```python
from build123d import *

# Parameters (mm, degrees)
SKETCH1_W           = 195.38
SKETCH1_H           = 100
BOSS_EXTRUDE1_DEPTH = 3
SKETCH2_R           = 2.75
CUT_EXTRUDE1_DEPTH  = 4
SKETCH3_R           = 2.75
SKETCH3_R_2         = 14.5
CUT_EXTRUDE2_DEPTH  = 4


with BuildPart() as part:
    # Sketch1 → Boss-Extrude1 (new body)
    with BuildSketch(Plane(origin=(0, 0, 0), x_dir=(1, 0, 0), z_dir=(0, 1, 0))):
        with Locations((97.69, -50)):
            Rectangle(SKETCH1_W, SKETCH1_H)
    extrude(amount=BOSS_EXTRUDE1_DEPTH)

    # Sketch2 → Cut-Extrude1 (cut, through all)
    with BuildSketch(Plane(origin=(0, 3, 0), x_dir=(1, 0, 0), z_dir=(0, 1, 0))):
        with Locations((185.38, -10)):
            Circle(SKETCH2_R)
        with Locations((185.38, -90)):
            Circle(SKETCH2_R)
        with Locations((10, -90)):
            Circle(SKETCH2_R)
        with Locations((10, -10)):
            Circle(SKETCH2_R)
    extrude(amount=-CUT_EXTRUDE1_DEPTH, mode=Mode.SUBTRACT)

    # Sketch3 → Cut-Extrude2 (cut, through all)
    with BuildSketch(Plane(origin=(0, 3, 0), x_dir=(1, 0, 0), z_dir=(0, 1, 0))):
        with Locations((90.316911264, -26.256219724)):
            Circle(SKETCH3_R)
        with Locations((72.212744361, -33.338953579)):
            Circle(SKETCH3_R)
        with Locations((64.419414315, -51.148781901)):
            Circle(SKETCH3_R)
        with Locations((115.209473441, -52.153716673)):
            Circle(SKETCH3_R)
        with Locations((107.416143395, -69.963544996)):
            Circle(SKETCH3_R)
        with Locations((89.311976492, -77.046278851)):
            Circle(SKETCH3_R)
        with Locations((71.50214817, -69.252948804)):
            Circle(SKETCH3_R)
        with Locations((89.814443878, -51.651249287)):
            Circle(SKETCH3_R_2)
    extrude(amount=-CUT_EXTRUDE2_DEPTH, mode=Mode.SUBTRACT)


solid = part.part
```
Check sheet for the modelled part. Datum: model origin and axes. Units: mm. Round coordinates to 2 decimals unless told otherwise and drop trailing zeros. Order: outer loops, then holes, each group sorted by start corner. A loop starts at its lowest first (then second) coordinate and runs counter-clockwise, first axis right, second up. Notation, with made-up numbers: (15.5, -14.5) - (63.5, -14.5) arc R19 ccw to (63.5, 2.5) - close; hole circle Ø3 at (83, 53). An arc over 180 degrees is marked (long way). Answer as CSV lines item,"result". Start each with the question number.
1) Section check C-C (y = 0.45). Give the number of separate pieces and of enclosed holes in the cut face, then the cut area to 3 significant figures.
2) Draft check along X on faces 1 (the face through (96, 3, 38)), 2 (the face through (9.404, 1.521, 92.685)). Enter one of: +X half, -X half, draft (parallel to the pull), parting line (faces both ways), or undercut.
3) Section check A-A (x = 10). Record the cut outline in (y, z), then the cut area to 3 significant figures.
4) Section check B-B (z = 90). Record the cut outline in (x, y), then the cut area to 3 significant figures.
5) Depth check by flat-ended pin: pin 1 (3.5 mm diameter, centred on x = 185.38, z = 10, fed in from +Y). Enter the tip coordinate at first touch or a pass-through.
6) Scan lines: probe 1 along X at (y, z) = (0.95, 10); probe 2 along Z at (x, y) = (185.38, 2); probe 3 along Z at (x, y) = (72.5, 0.5). Record each from-to range of solid material in increasing order.
Determined:
1,separate pieces,"1"
1,enclosed holes,"12"
1,area,"18,600 mm^2"
2,face 1,"draft"
2,face 2,"undercut"
3,outline,"(0, 0) - (3, 0) - (3, 7.25) - (0, 7.25) - close; (0, 12.75) - (3, 12.75) - (3, 87.25) - (0, 87.25) - close; (0, 92.75) - (3, 92.75) - (3, 100) - (0, 100) - close"
3,area,"267 mm^2"
4,outline,"(0, 0) - (7.25, 0) - (7.25, 3) - (0, 3) - close; (12.75, 0) - (182.63, 0) - (182.63, 3) - (12.75, 3) - close; (188.13, 0) - (195.38, 0) - (195.38, 3) - (188.13, 3) - close"
4,area,"553 mm^2"
5,pin 1,"through"
6,probe 1,"0 to 7.25, 12.75 to 182.63, 188.13 to 195.38"
6,probe 2,"0 to 7.25, 12.75 to 87.25, 92.75 to 100"
6,probe 3,"0 to 30.6, 36.07 to 66.69, 71.82 to 100"
